from build123d import *

# Parameters (mm, degrees)
SKETCH_1_W               = 48
SKETCH_1_H               = 26
ENCLOSURE_DEPTH          = 14
FILLET_2_R               = 2
SHELL_1_T                = -1.5
SKETCH_2_R               = 3
CABLE_ENTRY_DEPTH        = 57.356011214
SKETCH_3_R               = 4
CABLE_ENTRY_RELIEF_DEPTH = 1.6


with BuildPart() as part:
    # 草图1 → Enclosure (new body)
    with BuildSketch(Plane.XY):
        with Locations((24, 13)):
            Rectangle(SKETCH_1_W, SKETCH_1_H)
    extrude(amount=ENCLOSURE_DEPTH)

    # Fillet 2
    fillet_2_edges = [part.edges().sort_by_distance(p)[0] for p in [
        (0, 26, 7),
        (48, 26, 7),
        (48, 0, 7),
        (0, 0, 7),
    ]]
    fillet(fillet_2_edges, radius=FILLET_2_R)

    # 抽壳1
    shell_1_openings = [part.faces().sort_by_distance(p)[0] for p in [
        (24, 13, 14),
    ]]
    offset(amount=SHELL_1_T, openings=shell_1_openings, kind=Kind.INTERSECTION)

    # 草图2 → Cable_entry (cut, through all)
    with BuildSketch(Plane.XZ):
        with Locations(Location((24, 8, 0), (0, 0, 270))):
            Circle(SKETCH_2_R)
    extrude(amount=-CABLE_ENTRY_DEPTH, mode=Mode.SUBTRACT)

    # 草图3 → Cable_entry_relief (cut)
    with BuildSketch(Plane.XZ):
        with Locations(Location((24, 8, 0), (0, 0, 270))):
            Circle(SKETCH_3_R)
    extrude(amount=-CABLE_ENTRY_RELIEF_DEPTH, mode=Mode.SUBTRACT)


solid = part.part
Geometry check sheet. Reference: the model listing, model coordinates, mm. A direction names the side the tool comes from. Give positions to 0.01 mm unless a question says otherwise; leave off trailing zeros. Loops run counter-clockwise (first coordinate to the right, second up) from the corner with the lowest first, then second, coordinate; pieces in that order, holes last. Notation, with made-up numbers: (-31, 8.5) -> (20, 8.5) arc R23 cw to (20, 25.5) -> close; hole circle Ø7 at (49, 63.5). An arc over 180 degrees is marked (long way). Answer in a Markdown table with one row per item. Add a question column.
1) Cross-section at C-C on z = 2.5. Record the boundary of the cut face in (x, y), and give its area (3 significant figures).
2) Gauge pin test, flat end, axial feed: P1, Ø5, axis at x = 24, z = 8, coming from the +Y side. Record the tip position at first contact, or that the pin passes through.
3) Material ranges on probe 1 along X at (y, z) = (8.75, 7.25); probe 2 along Y at (x, z) = (11.5, 13.25); probe 3 along X at (y, z) = (25.7, 8), recorded low to high. Write a range as from..to.
4) Draft check along Y on faces 1 (the face through (24, 1.5, 3)), 2 (the face through (0.57, 0.6, 7.1)), 3 (the face through (24.9, 25.24, 5.14)). Enter one of: pulls with the +Y half, pulls with the -Y half, needs draft (parallel to the pull), parting line crosses it, or undercut.
5) Cross-section at B-B on x = 24. Record the boundary of the cut face in (y, z).
6) Cross-section at D-D on y = 4. Record the boundary of the cut face in (x, z).
7) Cross-section at A-A on z = 8. Record the boundary of the cut face in (x, y), and give its area (3 significant figures).
8) Set-up check for faces 4 (the face through (27.966, 0.74, 8.521)), 5 (the face through (23.7, 0, 3.8)), 6 (the face through (46.5, 13, 8)): record each of +Z, -Z, +X, -X, +Y, -Y from which the full face is reachable in a straight line by a thin tool's end or side.
Outcome:
| question | item | result |
|---|---|---|
| 1 | outline | (0, 2) arc R2 ccw to (2, 0) -> (46, 0) arc R2 ccw to (48, 2) -> (48, 24) arc R2 ccw to (46, 26) -> (2, 26) arc R2 ccw to (0, 24) -> close; hole (1.5, 2) arc R0.5 ccw to (2, 1.5) -> (46, 1.5) arc R0.5 ccw to (46.5, 2) -> (46.5, 24) arc R0.5 ccw to (46, 24.5) -> (2, 24.5) arc R0.5 ccw to (1.5, 24) -> close |
| 1 | area | 210 mm^2 |
| 2 | P1 | passes through |
| 3 | probe 1 | x = 0..1.5, 46.5..48 |
| 3 | probe 2 | y = 0..1.5, 24.5..26 |
| 3 | probe 3 | x = 0.95..21, 27..47.05 |
| 4 | face 1 | undercut |
| 4 | face 2 | pulls with the -Y half |
| 4 | face 3 | needs draft |
| 5 | outline | (0, 0) -> (26, 0) -> (26, 5) -> (24.5, 5) -> (24.5, 1.5) -> (1.5, 1.5) -> (1.5, 4) -> (0, 4) -> close; (0, 12) -> (1.5, 12) -> (1.5, 14) -> (0, 14) -> close; (24.5, 11) -> (26, 11) -> (26, 14) -> (24.5, 14) -> close |
| 6 | outline | (0, 0) -> (48, 0) -> (48, 14) -> (46.5, 14) -> (46.5, 1.5) -> (1.5, 1.5) -> (1.5, 14) -> (0, 14) -> close |
| 7 | outline | (0, 2) arc R2 ccw to (2, 0) -> (20, 0) -> (20, 1.5) -> (2, 1.5) arc R0.5 cw to (1.5, 2) -> (1.5, 24) arc R0.5 cw to (2, 24.5) -> (21, 24.5) -> (21, 26) -> (2, 26) arc R2 ccw to (0, 24) -> close; (27, 24.5) -> (46, 24.5) arc R0.5 cw to (46.5, 24) -> (46.5, 2) arc R0.5 cw to (46, 1.5) -> (28, 1.5) -> (28, 0) -> (46, 0) arc R2 ccw to (48, 2) -> (48, 24) arc R2 ccw to (46, 26) -> (27, 26) -> close |
| 7 | area | 189 mm^2 |
| 8 | face 4 | -Y |
| 8 | face 5 | +Z, -Z, +X, -X, -Y |
| 8 | face 6 | +Z |
